Here's the drawing with two shaded views (mm, measured from the low corner). I have some questions. A direction names the side the tool comes from. Coordinates: 2 decimals unless noted, no trailing zeros. Order: outer loops, then holes, each group sorted by start corner. A loop starts at its lowest first (then second) coordinate and runs counter-clockwise, first axis right, second up. Notation, with made-up numbers: (-9, 10.5) - (3, 10.5) arc R15 ccw to (3, 26.5) - close; hole circle Ø3 at (76, 32). An arc over 180 degrees is marked (long way). Answer as a JSON object with one key per item and string values. Group by question number.
(1) Imagine slicing it at D-D, the plane y = 8.25. Give the number of separate pieces and of enclosed holes in the cut face, and give its area (3 significant figures).
(2) Imagine slicing it at B-B, the plane y = 4. Write out the boundary of the cut face in (x, z).
(3) Which directions (+Z, -Z, +X, -X, +Y, -Y) give clear straight access to the entire face, cutting with the end or side of a thin tool? Please do the marked faces 1 and 2.
(4) Will this pin go through, and if not, where does the flat tip stop? P1, Ø12.5, axis at x = 14.5, z = 12, coming from the -Y side.
(5) Imagine slicing it at A-A, the plane z = 19.1. Write out the boundary of the cut face in (x, y).
(6) Please list where these lines run through material, in increasing order: probe 1 along Z at (x, y) = (12.6, 6.4); probe 2 along Y at (x, z) = (4.6, 2.2); probe 3 along Z at (x, y) = (20.6, 6.95).
(7) Imagine slicing it at C-C, the plane x = 12.6. Write out the boundary of the cut face in (y, z), and give its area (3 significant figures).
(8) We'd pull the mould along Z, two halves only. Please class the marked faces 3, 4 and 5: pulls with the +Z half, pulls with the -Z half, needs draft (parallel to the pull), parting line crosses it, or undercut.
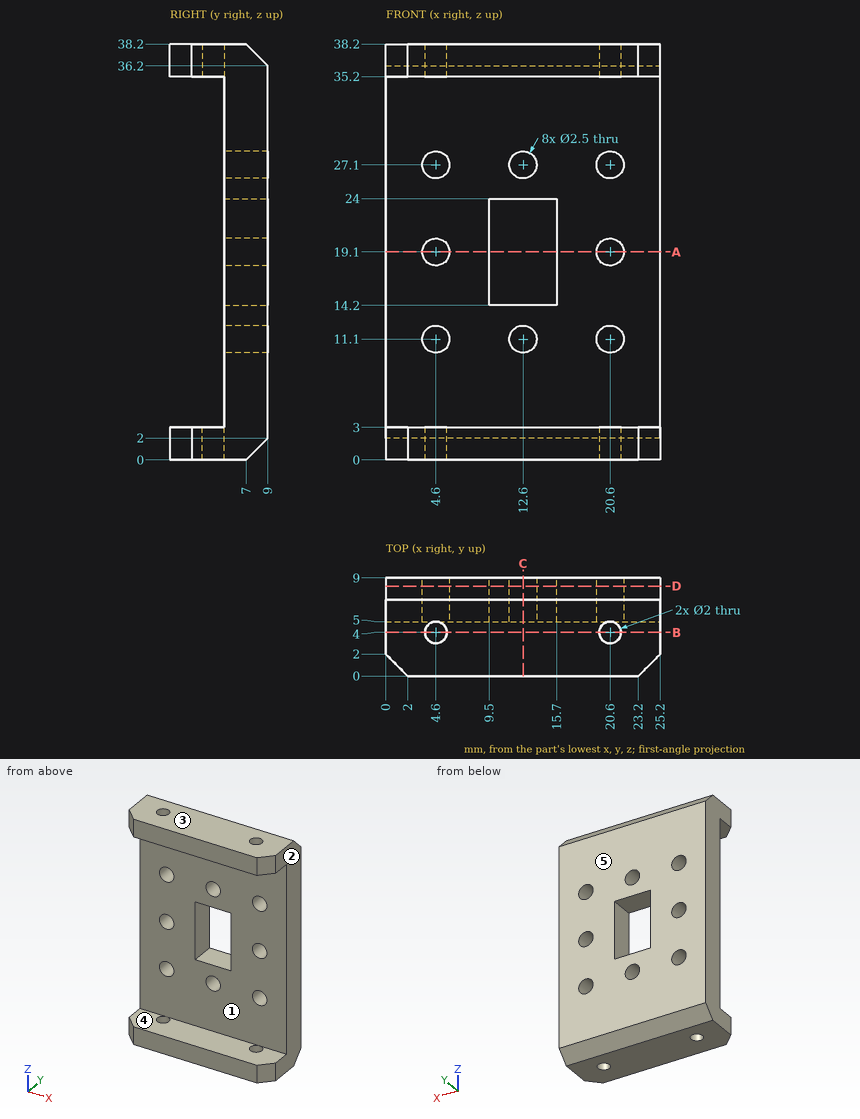
Result set:
{
 "1": {"separate pieces": "1", "enclosed holes": "9", "area": "800 mm^2"},
 "2": {"outline": "(0, 0) - (3.6, 0) - (3.6, 3) - (0, 3) - close; (0, 35.2) - (3.6, 35.2) - (3.6, 38.2) - (0, 38.2) - close; (5.6, 0) - (19.6, 0) - (19.6, 3) - (5.6, 3) - close; (5.6, 35.2) - (19.6, 35.2) - (19.6, 38.2) - (5.6, 38.2) - close; (21.6, 0) - (25.2, 0) - (25.2, 3) - (21.6, 3) - close; (21.6, 35.2) - (25.2, 35.2) - (25.2, 38.2) - (21.6, 38.2) - close"},
 "3": {"face 1": "+X, -X, -Y", "face 2": "+Z, -Z, +X, +Y, -Y"},
 "4": {"P1": "stops at y = 5"},
 "5": {"outline": "(0, 5) - (3.35, 5) - (3.35, 9) - (0, 9) - close; (5.85, 5) - (9.5, 5) - (9.5, 9) - (5.85, 9) - close; (15.7, 5) - (19.35, 5) - (19.35, 9) - (15.7, 9) - close; (21.85, 5) - (25.2, 5) - (25.2, 9) - (21.85, 9) - close"},
 "6": {"probe 1": "z = 0 to 9.85, 12.35 to 14.2, 24 to 25.85, 28.35 to 38.2", "probe 2": "y = 0 to 3, 5 to 9", "probe 3": "z = 0 to 9.85, 12.35 to 17.85, 20.35 to 25.85, 28.35 to 38.2"},
 "7": {"outline": "(0, 0) - (7, 0) - (9, 2) - (9, 9.85) - (5, 9.85) - (5, 3) - (0, 3) - close; (0, 35.2) - (5, 35.2) - (5, 28.35) - (9, 28.35) - (9, 36.2) - (7, 38.2) - (0, 38.2) - close; (5, 12.35) - (9, 12.35) - (9, 14.2) - (5, 14.2) - close; (5, 24) - (9, 24) - (9, 25.85) - (5, 25.85) - close", "area": "120 mm^2"},
 "8": {"face 3": "pulls with the +Z half", "face 4": "undercut", "face 5": "needs draft"}
}
